```python
from build123d import *

# Parameters (mm, degrees)
F1_DEPTH    = 5
F2_R        = 4
F3_DEPTH    = 25
F5_W        = 85
F5_H        = 8
F6_DEPTH    = 15
F7_T4_DEPTH = 371.701063592
F7_T9_DEPTH = 371.701063592
F8_SIZE     = 10


# Not quite as in the source:
# - a fillet or chamfer that OpenCascade refuses, or shapes differently, is made with other operations: its cross-section is extruded or revolved along the edge and cut away or added
# - a feature names something its author has since deleted; it is built from what else it names


with BuildPart() as f1:
    # F0 (on Top) → F1 (new body)
    with BuildSketch(Plane.XY):
        with BuildLine():
            ThreePointArc((-19.3933982822, 40.6066017178), (-16.1418070123, 35.7402514855), (-15, 30))
            ThreePointArc((-15, 30), (-30, 15), (-45, 30))
            Line((-45, 30), (-45, -30))
            ThreePointArc((-45, -30), (-30, -15), (-15, -30))
            ThreePointArc((-15, -30), (-16.1418070123, -35.7402514855), (-19.3933982822, -40.6066017178))
            ThreePointArc((-19.3933982822, -40.6066017178), (-1.9551429216, -35.9702766297), (14.3933982822, -43.6066017178))
            ThreePointArc((14.3933982822, -43.6066017178), (19.2597485145, -19.1418070123), (40, -33))
            Line((40, -33), (40, 33))
            ThreePointArc((40, 33), (19.2597485145, 19.1418070123), (14.3933982822, 43.6066017178))
            ThreePointArc((14.3933982822, 43.6066017178), (-1.9551429216, 35.9702766297), (-19.3933982822, 40.6066017178))
        make_face()
        with BuildLine():
            ThreePointArc((-15, -30), (-30, -15), (-45, -30))
            ThreePointArc((-45, -30), (-35.7402514855, -43.8581929877), (-19.3933982822, -40.6066017178))
            ThreePointArc((-19.3933982822, -40.6066017178), (-16.1418070123, -35.7402514855), (-15, -30))
        make_face()
        with BuildLine():
            ThreePointArc((-45, 30), (-30, 15), (-15, 30))
            ThreePointArc((-15, 30), (-16.1418070123, 35.7402514855), (-19.3933982822, 40.6066017178))
            ThreePointArc((-19.3933982822, 40.6066017178), (-35.7402514855, 43.8581929877), (-45, 30))
        make_face()
        with BuildLine():
            ThreePointArc((40, 33), (30.7402514855, 46.8581929877), (14.3933982822, 43.6066017178))
            ThreePointArc((14.3933982822, 43.6066017178), (19.2597485145, 19.1418070123), (40, 33))
        make_face()
        with BuildLine():
            ThreePointArc((14.3933982822, -43.6066017178), (30.7402514855, -46.8581929877), (40, -33))
            ThreePointArc((40, -33), (19.2597485145, -19.1418070123), (14.3933982822, -43.6066017178))
        make_face()
    extrude(amount=F1_DEPTH)


with BuildPart() as f3:
    # F2 (on Top) → F3 (new body)
    with BuildSketch(Plane.XY):
        with Locations((-30, 30)):
            Circle(F2_R)
    extrude(amount=F3_DEPTH)


with BuildPart() as f3b:
    # F2 (on Top) → F3, piece 2 (new body)
    with BuildSketch(Plane.XY):
        with Locations((25, 33)):
            Circle(F2_R)
    extrude(amount=F3_DEPTH)


with BuildPart() as f3c:
    # F2 (on Top) → F3, piece 3 (new body)
    with BuildSketch(Plane.XY):
        with Locations((25, -33)):
            Circle(F2_R)
    extrude(amount=F3_DEPTH)


with BuildPart() as f3d:
    # F2 (on Top) → F3, piece 4 (new body)
    with BuildSketch(Plane.XY):
        with Locations((-30, -30)):
            Circle(F2_R)
    extrude(amount=F3_DEPTH)


with BuildPart() as f1_1:
    add(f1.part)

    # F4: cut F3, F3b, F3c, F3d
    add(f3.part, mode=Mode.SUBTRACT)
    add(f3b.part, mode=Mode.SUBTRACT)
    add(f3c.part, mode=Mode.SUBTRACT)
    add(f3d.part, mode=Mode.SUBTRACT)

    # F5 (on Top) → F6 (join)
    with BuildSketch(Plane.XY):
        with Locations((-2.5, 16)):
            Rectangle(F5_W, F5_H)
        with Locations((-2.5, -16)):
            Rectangle(F5_W, F5_H)
    extrude(amount=F6_DEPTH)

    # F7: chamfer of 15 x 70 on 2 edges, made by hand


with BuildPart() as f7_tool2:
    # F7_s3 → F7_t4 (new body)
    with BuildSketch(Plane.XZ.offset(169.850531796)):
        Polygon((-30, 15), (40, 0), (40, 15), align=None)
    extrude(amount=-F7_T4_DEPTH)

    split(bisect_by=Plane.XY.offset(5), keep=Keep.TOP)


with BuildPart() as f1_2:
    add(f1_1.part)

    # F7_t1: cut F7_tool2
    add(f7_tool2.part, mode=Mode.SUBTRACT)


with BuildPart() as f7_tool7:
    # F7_s8 → F7_t9 (new body)
    with BuildSketch(Plane.XZ.offset(201.850531796)):
        Polygon((-30, 15), (40, 0), (40, 15), align=None)
    extrude(amount=-F7_T9_DEPTH)

    split(bisect_by=Plane.XY.offset(5), keep=Keep.TOP)


with BuildPart() as f1_3:
    add(f1_2.part)

    # F7_t6: cut F7_tool7
    add(f7_tool7.part, mode=Mode.SUBTRACT)

    # F8
    f8_edges = [f1_3.edges().sort_by_distance(p)[0] for p in [
        (-45, 16, 15),
        (-45, -16, 15),
    ]]
    chamfer(f8_edges, length=F8_SIZE)


solid = f1_3.part
```
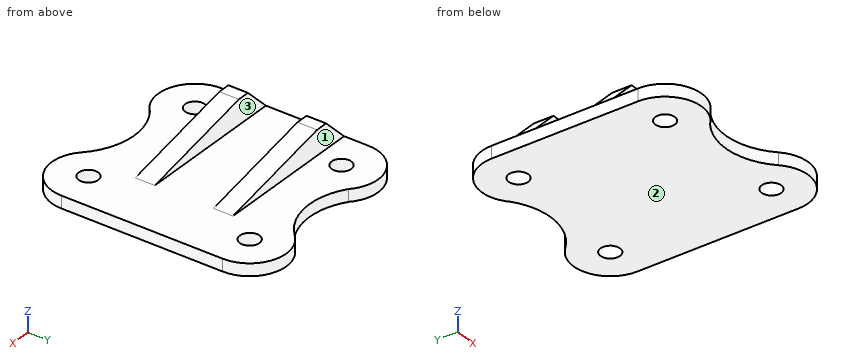
Verification items for the finished model (mm, model axes). Face numbers are marked on the shaded views. Coordinates: 2 decimals unless noted, no trailing zeros. Write each loop counter-clockwise with the first axis right and the second up, starting at its lowest first coordinate (ties: lowest second). Pieces come first, ordered by that corner, then holes. Notation, with made-up numbers: M 45,15 L 99,15 A21 ccw 99,26 Z; hole C -25,-1.75 d3. An arc over 180 degrees is marked long. Answer as a JSON object with one key per item and string values. Group by question number.
(1) Cross-section at C-C, the plane x = -14. Record the cut outline in (y, z).
(2) Cross-section at A-A, the plane z = 12. Record the cut outline in (x, y).
(3) Cross-section at D-D, the plane z = 2.75. Record the cut outline in (x, y), and give its area (3 significant figures).
(4) Gauge pin test, flat ends, axial feed: pin 1 (4 mm diameter, centred on x = -22.5, z = 12, fed in from -Y); pin 2 (8 mm diameter, centred on x = -29, z = 11.5, fed in from +Y); pin 3 (6 mm diameter, centred on x = -28, z = 3.5, fed in from -Y). Record the tip position at first contact, or that the pin passes through.
(5) Cross-section at B-B, the plane x = 25. Record the cut outline in (y, z), and give its area (3 significant figures).
(6) Material ranges on line 1 (Y direction, x = -30, z = 1.3); line 2 (Y direction, x = -36, z = 5.25); line 3 (X direction, y = -33, z = 1.35), recorded low to high.
(7) Release check for a two-part mould opening along Y. For the marked faces 1, 2 and 3 record: +Y half, -Y half, draft (parallel to the pull), parting line (faces both ways), or undercut.
Reply:
{
 "1": {"outline": "M -37.71,0 L 37.71,0 L 37.71,5 L 20,5 L 20,11.57 L 12,11.57 L 12,5 L -12,5 L -12,11.57 L -20,11.57 L -20,5 L -37.71,5 Z"},
 "2": {"outline": "M -38,-20 L -16,-20 L -16,-12 L -38,-12 Z; M -38,12 L -16,12 L -16,20 L -38,20 Z"},
 "3": {"outline": "M -45,-30 A15 ccw -19.39,-40.61 A26.43 cw 14.39,-43.61 A15 ccw 40,-33 L 40,33 A15 ccw 14.39,43.61 A26.43 cw -19.39,40.61 A15 ccw -45,30 Z; hole C -30,-30 d8; hole C -30,30 d8; hole C 25,-33 d8; hole C 25,33 d8", "area": "6,870 mm²"},
 "4": {"pin 1": "y = -20", "pin 2": "y = 20", "pin 3": "y = -45"},
 "5": {"outline": "M -48,0 L -37,0 L -37,5 L -48,5 Z; M -29,0 L 29,0 L 29,5 L -29,5 Z; M 37,0 L 48,0 L 48,5 L 37,5 Z", "area": "400 mm²"},
 "6": {"line 1": "-45 to -34, -26 to 26, 34 to 45", "line 2": "-20 to -12, 12 to 20", "line 3": "-44.7 to -32.65, -27.35 to 21, 29 to 40"},
 "7": {"face 1": "+Y half", "face 2": "draft", "face 3": "undercut"}
}
